Read the model definition and answer for the solid it produces. Units are mm, in the model's axes. Give positions to 0.01 mm unless a question says otherwise; leave off trailing zeros. Order: outer loops, then holes, each group sorted by start corner. A loop starts at its lowest first (then second) coordinate and runs counter-clockwise, first axis right, second up. Notation, with made-up numbers: (-13.5, 27.5) - (2.5, 27.5) arc R12 cw to (2.5, 32.5) - close; hole circle Ø6 at (5, 62.5). An arc over 180 degrees is marked (long way). Write each question's results on one line, items separated by ' | '.
from build123d import *


with BuildPart() as part:
    # Sketch1 → Revolve1 (revolve)
    with BuildSketch(Plane(origin=(0, 0, 0), x_dir=(0, 0, -1), z_dir=(1, 0, 0))):
        with BuildLine():
            Line((0, 0), (-50.959835356, 0))
            Line((-50.959835356, 0), (-61.054255014, 0))
            Line((-61.054255014, 0), (-61.054255014, 30.599788402))
            Line((-61.054255014, 30.599788402), (-60.054255014, 30))
            Line((-60.054255014, 30), (-30.054255014, 29.5))
            ThreePointArc((-30.054255014, 29.5), (-27.754838856, 29.797720054), (-25.637373582, 30.742332522))
            ThreePointArc((-25.637373582, 30.742332522), (-22.902920152, 32.314145749), (-20.042663952, 33.643343571))
            ThreePointArc((-20.042663952, 33.643343571), (-10.179122164, 36.1760026), (0, 35.877187771))
            Line((0, 35.877187771), (0, 34.862194457))
            Line((0, 34.862194457), (0, 0))
        make_face()
    revolve(axis=Axis((0, 0, 0), (0, 0, 1)))


solid = part.part
(1) The mould has two halves that part along Z. Classify faces 1 (the face through (0, 0, 61.054)), 2 (the face through (-1, -1, 0)), 3 (the face through (-8.94, 28.37, 44.84)): pulls with the +Z half, pulls with the -Z half, needs draft (parallel to the pull), parting line crosses it, or undercut.
Conclusion:
face 1: pulls with the +Z half | face 2: pulls with the -Z half | face 3: undercut
(2) Section A-A (z = 19) is taken. Give the vertices of the cut face in (x, y), plus the area to 3 significant figures.
Conclusion:
outline: circle Ø68.11 at (0, 0) | area: 3,640 mm^2
(3) Each of these flat-tipped pins is pushed along its axis until it touches: pin 1 (1.5 mm diameter, centred on y = -14, z = 13.5, fed in from -X); pin 2 (5 mm diameter, centred on x = 17.5, z = 43, fed in from -Y); pin 3 (4 mm diameter, centred on y = 14, z = 14.5, fed in from +X). Where does it stop, or does it pass through?
Conclusion:
pin 1: x = -33.14 | pin 2: y = -25.65 | pin 3: x = 33.47
(4) Section B-B (z = 51) is taken. Give the vertices of the cut face in (x, y), plus the area to 3 significant figures.
Conclusion:
outline: circle Ø59.7 at (0, 0) | area: 2,800 mm^2
(5) Consider probe 1 along X at (y, z) = (-19.5, 18); probe 2 along Z at (x, y) = (-22, 25); probe 3 along Y at (x, z) = (-22.5, 24.5). Determine where each line is inside the solid, lowest interval first. Write a range as [from, to].
Conclusion:
probe 1: [-28.36, 28.36] | probe 2: [0, 20.84] | probe 3: [-21.95, 21.95]
